```python
from build123d import *

# Parameters (mm, degrees)
SKETCH_W        = 88
SKETCH_H        = 42
PAD_DEPTH       = 40
SKETCH001_W     = 80
SKETCH001_H     = 42.719318
POCKET_DEPTH    = 36
SKETCH002_R     = 14
POCKET001_DEPTH = 5
SKETCH003_W     = 20
SKETCH003_H     = 4
PAD001_DEPTH    = 80
SKETCH004_R     = 2.25
POCKET002_DEPTH = 5
POCKET003_DEPTH = 88.001
FILLET_R        = 3


with BuildPart() as part:
    # Sketch → Pad (new body)
    with BuildSketch(Plane.XY):
        with Locations((0, 17)):
            Rectangle(SKETCH_W, SKETCH_H)
    extrude(amount=PAD_DEPTH)

    # Sketch001 → Pocket (cut)
    with BuildSketch(Plane(origin=(0, 0, 0), x_dir=(1, 0, 0), z_dir=(0, 0, -1))):
        with Locations((0, -21.359659)):
            Rectangle(SKETCH001_W, SKETCH001_H)
    extrude(amount=-POCKET_DEPTH, mode=Mode.SUBTRACT)

    # Sketch002 → Pocket001 (cut)
    with BuildSketch(Plane.XY.offset(40)):
        with Locations((-22, 19)):
            Circle(SKETCH002_R)
        with Locations((22, 19)):
            Circle(SKETCH002_R)
    extrude(amount=-POCKET001_DEPTH, mode=Mode.SUBTRACT)

    # Sketch003 → Pad001 (new body)
    with BuildSketch(Plane(origin=(40, 0, 0), x_dir=(0, -1, 0), z_dir=(-1, 0, 0))):
        with Locations((-10, 2)):
            Rectangle(SKETCH003_W, SKETCH003_H)
    extrude(amount=PAD001_DEPTH)

    # Sketch004 → Pocket002 (cut)
    with BuildSketch(Plane(origin=(0, 0, 0), x_dir=(1, 0, 0), z_dir=(0, 0, -1))):
        with Locations((-22, -10)):
            Circle(SKETCH004_R)
        with Locations((22, -10)):
            Circle(SKETCH004_R)
    extrude(amount=-POCKET002_DEPTH, mode=Mode.SUBTRACT)

    # Sketch006 → Pocket003 (cut, through all)
    with BuildSketch(Plane.YZ.offset(44)):
        Polygon((20, 0), (38, 36), (38, 0), align=None)
    extrude(amount=-POCKET003_DEPTH, mode=Mode.SUBTRACT)

    # Fillet
    fillet_edges = [part.edges().sort_by_distance(p)[0] for p in [
        (-44, 17, 40),
        (0, 38, 40),
        (44, 17, 40),
        (0, -4, 40),
        (44, -4, 20),
        (-44, -4, 20),
        (44, 38, 38),
        (-44, 38, 38),
    ]]
    fillet(fillet_edges, radius=FILLET_R)


solid = part.part
```
The model under review builds one solid part; all positions refer to its coordinate system, in mm. A direction names the side the tool comes from. Round coordinates to 2 decimals unless told otherwise and drop trailing zeros. Order: outer loops, then holes, each group sorted by start corner. A loop starts at its lowest first (then second) coordinate and runs counter-clockwise, first axis right, second up. Notation, with made-up numbers: M 35,28.25 L 43,28.25 A27 cw 43,57.25 Z; hole C 34.25,37 d5. An arc over 180 degrees is marked long. Use a Markdown table: item, result.
1) Consider section A-A (x = 22). Write out the cut boundary in (y, z), then the cut area to 3 significant figures.
Report:
| item | result |
|---|---|
| outline | M -4,0 L 7.75,0 L 7.75,4 L 0,4 L 0,36 L 5,36 L 5,40 L -1,40 A3 ccw -4,37 Z; M 12.25,0 L 20,0 L 20,4 L 12.25,4 Z; M 33,36 L 38,36 L 38,37 A3 ccw 35,40 L 33,40 Z |
| area | 258 mm^2 |
2) Tool access review of faces 1 (the face through (1, 20, 2)), 2 (the face through (-20.79, 8.103, 1.972)), 3 (the face through (-1, 19, 36)), 4 (the face through (-15.5, 6.6, 38)): name each direction out of +Z, -Z, +X, -X, +Y, -Y from which nothing blocks a thin tool from reaching the whole face with its end or side.
Report:
| item | result |
|---|---|
| face 1 | -Z, +Y |
| face 2 | +Z, -Z |
| face 3 | +Y |
| face 4 | +Z |
3) Insertion check: pin 1 (9.5 mm diameter, centred on x = -18.5, z = 23.5, fed in from +Y); pin 2 (17 mm diameter, centred on x = 22, y = 19, fed in from +Z); pin 3 (6 mm diameter, centred on x = -26.5, y = 33, fed in from -Z); pin 4 (3.5 mm diameter, centred on x = -22, y = 10, fed in from -Z). Each pin has a flat end and moves straight along its axis. Give the tip position at first contact, or say it passes through.
Report:
| item | result |
|---|---|
| pin 1 | y = 0 |
| pin 2 | z = 4 |
| pin 3 | z = 36 |
| pin 4 | through |
4) Consider section D-D (z = 7). Write out the cut boundary in (x, y).
Report:
| item | result |
|---|---|
| outline | M -44,-1 A3 ccw -41,-4 L 41,-4 A3 ccw 44,-1 L 44,23.5 L 40,23.5 L 40,0 L -40,0 L -40,23.5 L -44,23.5 Z |
5) Consider section C-C (y = 19). Write out the cut boundary in (x, z).
Report:
| item | result |
|---|---|
| outline | M -44,0 L 44,0 L 44,37 A3 ccw 41,40 L 36,40 L 36,36 L 40,36 L 40,4 L -40,4 L -40,36 L -36,36 L -36,40 L -41,40 A3 ccw -44,37 Z; M -8,36 L 8,36 L 8,40 L -8,40 Z |
6) Wall thickness on line 1 along X through (y, z) = (11, 23); line 2 along X through (y, z) = (10, 2); line 3 along Z through (x, y) = (-35, 3): over which ranges is each line inside the solid? List them lowest first. Write a range as [from, to].
Report:
| item | result |
|---|---|
| line 1 | [-44, -40], [40, 44] |
| line 2 | [-44, -24.25], [-19.75, 19.75], [24.25, 44] |
| line 3 | [0, 4], [36, 40] |
7) Consider section B-B (z = 3). Write out the cut boundary in (x, y).
Report:
| item | result |
|---|---|
| outline | M -44,-1 A3 ccw -41,-4 L 41,-4 A3 ccw 44,-1 L 44,21.5 L 40,21.5 L 40,20 L -40,20 L -40,21.5 L -44,21.5 Z; hole C -22,10 d4.5; hole C 22,10 d4.5 |
8) Draft analysis for pull direction Z (two halves, no side actions). For faces 5 (the face through (40, 15, 22)), 6 (the face through (0.57, 37.14, 39.1)), 7 (the face through (1, 8, 0)), 8 (the face through (28.5, 6.6, 38)), state which applies: released by +Z, released by -Z, zero draft, split by the parting line, or undercut.
Report:
| item | result |
|---|---|
| face 5 | undercut |
| face 6 | released by +Z |
| face 7 | released by -Z |
| face 8 | zero draft |
